Design review of the part built by this model. Coordinates are the model's own, in mm. A direction names the side the tool comes from. Give positions to 0.01 mm unless a question says otherwise; leave off trailing zeros. Write each loop counter-clockwise with the first axis right and the second up, starting at its lowest first coordinate (ties: lowest second). Pieces come first, ordered by that corner, then holes.
```python
from build123d import *

# Parameters (mm, degrees)
F0_W     = 19.05
F0_H     = 34.925
F1_DEPTH = 6.35
F2_W     = 19.05
F2_H     = 6.35
F3_DEPTH = 31.75


with BuildPart() as f1:
    # F0 (on Front) → F1 (new body)
    with BuildSketch(Plane.XZ):
        with Locations((9.525, -17.4625)):
            Rectangle(F0_W, F0_H)
        with BuildLine():
            ThreePointArc((7.1374, -12.7), (9.525, -10.3124), (11.9126, -12.7))
            Line((11.9126, -12.7), (11.9126, -30.48))
            ThreePointArc((11.9126, -30.48), (9.525, -32.8676), (7.1374, -30.48))
            Line((7.1374, -30.48), (7.1374, -12.7))
        make_face(mode=Mode.SUBTRACT)
    extrude(amount=F1_DEPTH)

    # F2 (on face) → F3 (join)
    with BuildSketch(Plane(origin=(0, 0, 0), x_dir=(-1, 0, 0), z_dir=(0, 1, 0))):
        with Locations((-9.525, -3.175)):
            Rectangle(F2_W, F2_H)
    extrude(amount=F3_DEPTH)


solid = f1.part
```
(1) Clearance check with flat-ended pins moving along their axes: P1, Ø10, axis at x = 6, y = 22, coming from the -Z side; P2, Ø5.5, axis at x = 9, z = -19.5, coming from the +Y side. State where each tip first meets the part, or that it passes through.
Resolved:
P1: stops at z = -6.35
P2: stops at y = 0
(2) Consider section C-C, the plane x = 9. Give the boundary of the cut face in (y, z) (3 decimals), then the cut area to 3 significant figures.
Resolved:
outline: (-6.35, -34.925) - (0, -34.925) - (0, -32.809) - (-6.35, -32.809) - close; (-6.35, -10.371) - (0, -10.371) - (0, -6.35) - (31.75, -6.35) - (31.75, 0) - (-6.35, 0) - close
area: 281 mm2
(3) Consider section A-A, the plane z = -19.5. Give the boundary of the cut face in (x, y).
Resolved:
outline: (0, -6.35) - (7.14, -6.35) - (7.14, 0) - (0, 0) - close; (11.91, -6.35) - (19.05, -6.35) - (19.05, 0) - (11.91, 0) - close
(4) Consider section D-D, the plane x = 16.5. Give the boundary of the cut face in (y, z) (3 decimals), then the cut area to 3 significant figures.
Resolved:
outline: (-6.35, -34.925) - (0, -34.925) - (0, -6.35) - (31.75, -6.35) - (31.75, 0) - (-6.35, 0) - close
area: 423 mm2
(5) Tool access review of faces 1 (the face through (14, -6.35, -17)), 2 (the face through (14, 0, -20)), 3 (the face through (9.578, -3.131, -32.867)): name each direction out of +Z, -Z, +X, -X, +Y, -Y from which nothing blocks a thin tool from reaching the whole face with its end or side.
Resolved:
face 1: +Z, -Z, +X, -X, -Y
face 2: -Z, +X, -X, +Y
face 3: +Y, -Y
(6) To check wall thickness, follow L1, parallel to X at y = -4, z = -27.5; L2, parallel to Z at x = 4.5, y = 4. State the ranges of each line that lie inside material, in increasing order.
Resolved:
L1: x = 0 to 7.14, 11.91 to 19.05
L2: z = -6.35 to 0
(7) Consider section B-B, the plane y = -2. Give the boundary of the cut face in (x, z) (3 decimals), then the cut area to 3 significant figures.
Resolved:
outline: (0, -34.925) - (19.05, -34.925) - (19.05, 0) - (0, 0) - close; hole (7.137, -30.48) arc R2.388 ccw to (11.913, -30.48) - (11.913, -12.7) arc R2.388 ccw to (7.137, -12.7) - close
area: 563 mm2
(8) Mouldability with a two-part tool opening along Z and no side actions: class faces 4 (the face through (10, 12, 0)), 5 (the face through (7.137, -3, -22)), 6 (the face through (10, 16, -6.35)) as pulls with the +Z half, pulls with the -Z half, needs draft (parallel to the pull), parting line crosses it, or undercut.
Resolved:
face 4: pulls with the +Z half
face 5: undercut
face 6: pulls with the -Z half
